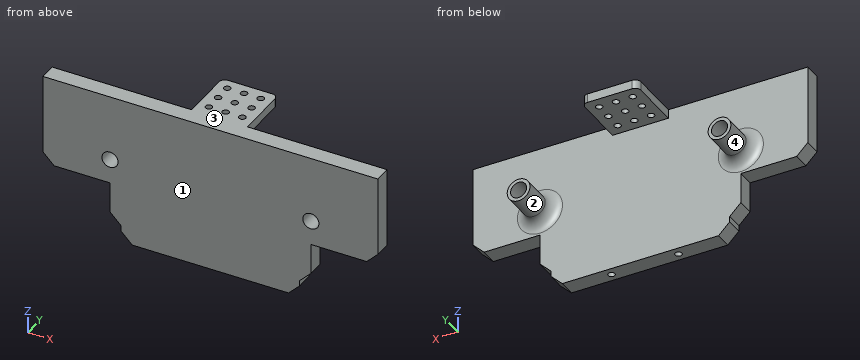
```python
from build123d import *

# Parameters (mm, degrees)
SKETCH1_W           = 150
SKETCH1_H           = 59.51
BOSS_EXTRUDE1_DEPTH = 7.5
SKETCH2_R           = 5.1
BOSS_EXTRUDE2_DEPTH = 17.5
FILLET1_R           = 5
SKETCH3_R           = 3.6
CUT_EXTRUDE1_DEPTH  = 25
SKETCH4_W           = 30
SKETCH4_H           = 7.5
CUT_EXTRUDE2_DEPTH  = 18.75
CHAMFER1_SIZE       = 5
SKETCH5_W           = 80
SKETCH5_H           = 7.5
BOSS_EXTRUDE3_DEPTH = 7.5
CHAMFER2_SIZE       = 5
SKETCH6_R           = 1.5
CUT_EXTRUDE3_DEPTH  = 7.5
SKETCH7_W           = 25
SKETCH7_H           = 4
BOSS_EXTRUDE4_DEPTH = 25
SKETCH8_R           = 1.5
CUT_EXTRUDE4_DEPTH  = 5
FILLET2_R           = 2.5


with BuildPart() as part:
    # Sketch1 → Boss-Extrude1 (new body)
    with BuildSketch(Plane(origin=(0, 0, 0), x_dir=(1, 0, 0), z_dir=(0, 1, 0))):
        Rectangle(SKETCH1_W, SKETCH1_H)
    extrude(amount=BOSS_EXTRUDE1_DEPTH)

    # Sketch2 → Boss-Extrude2 (add)
    with BuildSketch(Plane(origin=(0, 7.5, 0), x_dir=(1, 0, 0), z_dir=(0, 1, 0))):
        with Locations(Location((-45, 0, 0), (0, 0, 270))):
            Circle(SKETCH2_R)
        with Locations(Location((45, 0, 0), (0, 0, 270))):
            Circle(SKETCH2_R)
    extrude(amount=BOSS_EXTRUDE2_DEPTH)

    # Fillet1
    fillet1_edges = [part.edges().sort_by_distance(p)[0] for p in [
        (-45, 7.5, -5.1),
        (45, 7.5, -5.1),
    ]]
    fillet(fillet1_edges, radius=FILLET1_R)

    # Sketch3 → Cut-Extrude1 (cut)
    with BuildSketch(Plane(origin=(0, 25, 0), x_dir=(1, 0, 0), z_dir=(0, 1, 0))):
        with Locations(Location((-45, 0, 0), (0, 0, 270))):
            Circle(SKETCH3_R)
        with Locations(Location((45, 0, 0), (0, 0, 270))):
            Circle(SKETCH3_R)
    extrude(amount=-CUT_EXTRUDE1_DEPTH, mode=Mode.SUBTRACT)

    # Sketch4 → Cut-Extrude2 (cut)
    with BuildSketch(Plane(origin=(0, 0, -29.755), x_dir=(-1, 0, 0), z_dir=(0, 0, -1))):
        with Locations((-60, 3.75)):
            Rectangle(SKETCH4_W, SKETCH4_H)
        with Locations((60, 3.75)):
            Rectangle(SKETCH4_W, SKETCH4_H)
    extrude(amount=-CUT_EXTRUDE2_DEPTH, mode=Mode.SUBTRACT)

    # Chamfer1
    chamfer1_edges = [part.edges().sort_by_distance(p)[0] for p in [
        (75, 3.75, -11.005),
        (45, 3.75, -29.755),
        (-75, 3.75, -11.005),
        (-45, 3.75, -29.755),
    ]]
    chamfer(chamfer1_edges, length=CHAMFER1_SIZE)

    # Sketch5 → Boss-Extrude3 (add)
    with BuildSketch(Plane(origin=(0, 0, -29.755), x_dir=(-1, 0, 0), z_dir=(0, 0, -1))):
        with Locations((0, 3.75)):
            Rectangle(SKETCH5_W, SKETCH5_H)
    extrude(amount=BOSS_EXTRUDE3_DEPTH)

    # Chamfer2
    chamfer2_edges = [part.edges().sort_by_distance(p)[0] for p in [
        (40, 3.75, -37.255),
        (-40, 3.75, -37.255),
    ]]
    chamfer(chamfer2_edges, length=CHAMFER2_SIZE)

    # Sketch6 → Cut-Extrude3 (cut)
    with BuildSketch(Plane(origin=(0, 0, -37.255), x_dir=(-1, 0, 0), z_dir=(0, 0, -1))):
        with Locations((-15, 3.75)):
            Circle(SKETCH6_R)
        with Locations((15, 3.75)):
            Circle(SKETCH6_R)
    extrude(amount=-CUT_EXTRUDE3_DEPTH, mode=Mode.SUBTRACT)

    # Sketch7 → Boss-Extrude4 (add)
    with BuildSketch(Plane(origin=(0, 7.5, 0), x_dir=(1, 0, 0), z_dir=(0, 1, 0))):
        with Locations((0, -27.755)):
            Rectangle(SKETCH7_W, SKETCH7_H)
    extrude(amount=BOSS_EXTRUDE4_DEPTH)

    # Sketch8 → Cut-Extrude4 (cut)
    with BuildSketch(Plane(origin=(0, 0, 25.755), x_dir=(-1, 0, 0), z_dir=(0, 0, -1))):
        with Locations((-7.5, 20)):
            Circle(SKETCH8_R)
        with Locations((0, 20)):
            Circle(SKETCH8_R)
        with Locations((-7.5, 27.5)):
            Circle(SKETCH8_R)
        with Locations((0, 27.5)):
            Circle(SKETCH8_R)
        with Locations((7.5, 27.5)):
            Circle(SKETCH8_R)
        with Locations((7.5, 20)):
            Circle(SKETCH8_R)
        with Locations((-7.5, 12.5)):
            Circle(SKETCH8_R)
        with Locations((0, 12.5)):
            Circle(SKETCH8_R)
        with Locations((7.5, 12.5)):
            Circle(SKETCH8_R)
    extrude(amount=-CUT_EXTRUDE4_DEPTH, mode=Mode.SUBTRACT)

    # Fillet2
    fillet2_edges = [part.edges().sort_by_distance(p)[0] for p in [
        (-12.5, 32.5, 27.755),
        (12.5, 32.5, 27.755),
    ]]
    fillet(fillet2_edges, radius=FILLET2_R)


solid = part.part
```
Could you check a few things on this model? Use its own coordinates, in mm. Face numbers are marked on the shaded views. A direction names the side the tool comes from. Round coordinates to 2 decimals unless told otherwise and drop trailing zeros. Loops run counter-clockwise (first coordinate to the right, second up) from the corner with the lowest first, then second, coordinate; pieces in that order, holes last.
Q1. I want a section at D-D (x = -20.5). Write out the boundary of the cut face in (y, z) (3 decimals), and give its area (3 significant figures).
Q2. Please list where these lines run through material, in increasing order: L1, parallel to Y at x = 0, z = 28.7; L2, parallel to Y at x = 15, z = -34.25; L3, parallel to Y at x = -65, z = 6.5.
Q3. For P1, Ø4, axis at x = 56, y = 2.5, coming from the -Z side (3 decimals); P2, Ø1.5, axis at x = -15, y = 3.5, coming from the -Z side (3 decimals); P3, Ø8, axis at x = 46, z = 0, coming from the +Y side, each with a flat end and sliding along its axis, tell me the tip position at first contact or that it passes through.
Q4. On a 3-axis mill with a long thin cutter (end or side, diameter ignored), from which of +Z, -Z, +X, -X, +Y, -Y can I reach the whole of each face in a straight line? I mean the marked faces 1 and 2. Say none if no direction works.
Q5. I want a section at A-A (y = 20). Write out the boundary of the cut face in (x, z) (3 decimals), and give its area (3 significant figures).
Q6. I want a section at B-B (x = 15). Write out the boundary of the cut face in (y, z) (3 decimals).
Q7. Thinking about a two-plate mould opening in X: for the marked faces 3 and 4, which applies, pulls with the +X half, pulls with the -X half, needs draft (parallel to the pull), parting line crosses it, or undercut?
Q8. I want a section at C-C (z = -14.5). Write out the boundary of the cut face in (x, y).
Answer below:
1. outline: (0, -37.255) - (7.5, -37.255) - (7.5, 29.755) - (0, 29.755) - close
1. area: 503 mm2
2. L1: y = 0 to 11, 14 to 18.5, 21.5 to 26, 29 to 32.5
2. L2: y = 0 to 2.25, 5.25 to 7.5
2. L3: y = 0 to 7.5
3. P1: stops at z = -11.005
3. P2: stops at z = -29.755
3. P3: stops at y = 25
4. face 1: +Z, -Z, +X, -X, -Y
4. face 2: +Y
5. outline: circle Ø10.2 at (-45, 0); (-12.5, 25.755) - (-9, 25.755) - (-9, 29.755) - (-12.5, 29.755) - close; (-6, 25.755) - (-1.5, 25.755) - (-1.5, 29.755) - (-6, 29.755) - close; (1.5, 25.755) - (6, 25.755) - (6, 29.755) - (1.5, 29.755) - close; (9, 25.755) - (12.5, 25.755) - (12.5, 29.755) - (9, 29.755) - close; circle Ø10.2 at (45, 0); hole circle Ø7.2 at (-45, 0); hole circle Ø7.2 at (45, 0)
5. area: 146 mm2
6. outline: (0, -37.255) - (2.25, -37.255) - (2.25, -29.755) - (5.25, -29.755) - (5.25, -37.255) - (7.5, -37.255) - (7.5, 29.755) - (0, 29.755) - close
7. face 3: needs draft
7. face 4: undercut
8. outline: (-45, 0) - (45, 0) - (45, 7.5) - (-45, 7.5) - close
